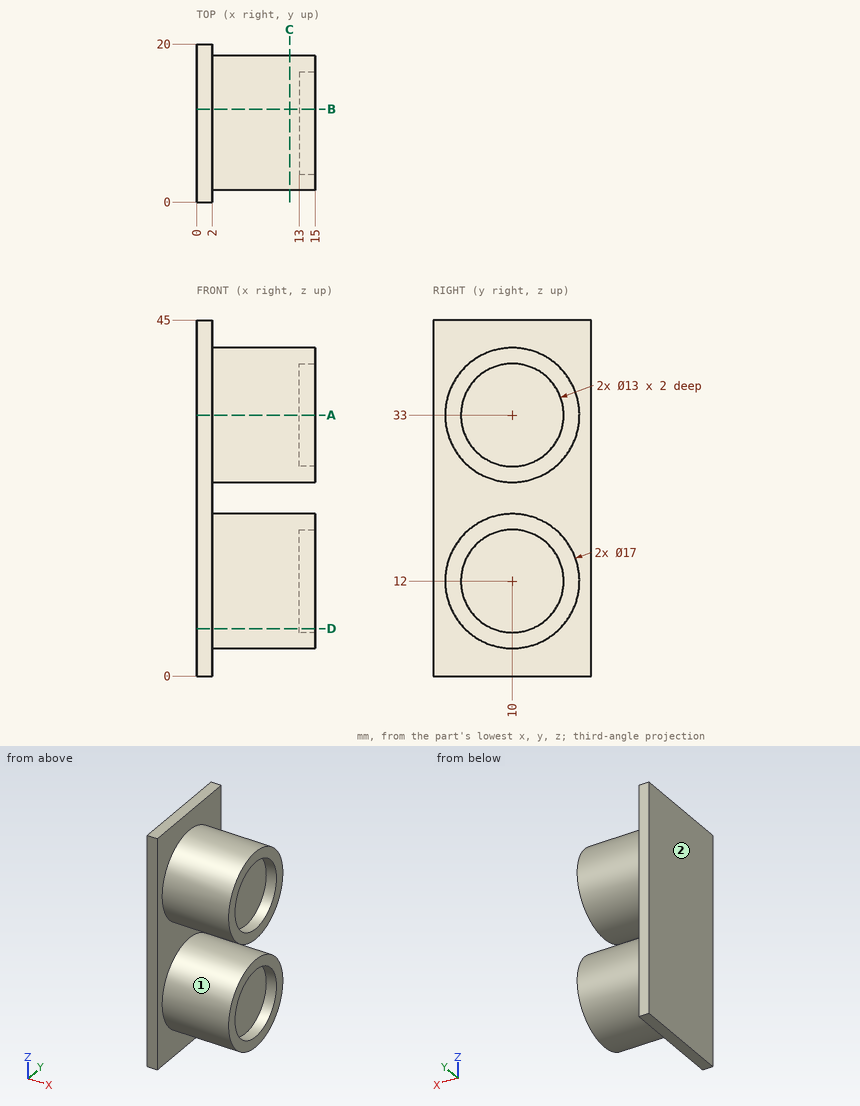
The drawing under review shows one solid part. Ordinate dimensions are in mm from its lowest x, y, z. Give positions to 0.01 mm unless a question says otherwise; leave off trailing zeros. Order: outer loops, then holes, each group sorted by start corner. A loop starts at its lowest first (then second) coordinate and runs counter-clockwise, first axis right, second up. Notation, with made-up numbers: (63, 53) - (84, 53) arc R19 ccw to (84, 78) - close; hole circle Ø11 at (78, 62). An arc over 180 degrees is marked (long way). Answer as a JSON object with one key per item and string values. Group by question number.
Item 1: Take a section at C-C on x = 11.75. Give the boundary of the cut face in (y, z).
Item 2: Wall thickness on line 1 along Y through (x, z) = (13.5, 33); line 2 along X through (y, z) = (11.5, 15.5); line 3 along Z through (x, y) = (7.5, 3.5): over which ranges is each line inside the solid? List them lowest first.
Item 3: Take a section at B-B on y = 11.75. Give the boundary of the cut face in (x, z).
Item 4: Draft analysis for pull direction Z (two halves, no side actions). For the marked faces 1 and 2, state which applies: pulls with the +Z half, pulls with the -Z half, needs draft (parallel to the pull), parting line crosses it, or undercut.
Item 5: Clearance check with flat-ended pins moving along their axes: pin 1 Ø4 at (y, z) = (11, 14.5) entering from +X; pin 2 Ø6 at (x, y) = (7, 14.5) entering from +Z; pin 3 Ø1.5 at (x, y) = (8.5, 10) entering from +Z. State where each tip first meets the part, or that it passes through.
Item 6: Take a section at A-A on z = 33. Give the boundary of the cut face in (x, y), and give its area (3 significant figures).
Item 7: Take a section at D-D on z = 6. Give the boundary of the cut face in (x, y).
Reported:
{
 "1": {"outline": "circle Ø17 at (10, 12); circle Ø17 at (10, 33)"},
 "2": {"line 1": "1.5 to 3.5, 16.5 to 18.5", "line 2": "0 to 13", "line 3": "6.52 to 17.48, 27.52 to 38.48"},
 "3": {"outline": "(0, 0) - (2, 0) - (2, 3.68) - (15, 3.68) - (15, 5.74) - (13, 5.74) - (13, 18.26) - (15, 18.26) - (15, 20.32) - (2, 20.32) - (2, 24.68) - (15, 24.68) - (15, 26.74) - (13, 26.74) - (13, 39.26) - (15, 39.26) - (15, 41.32) - (2, 41.32) - (2, 45) - (0, 45) - close"},
 "4": {"face 1": "undercut", "face 2": "needs draft"},
 "5": {"pin 1": "x = 13", "pin 2": "z = 41.37", "pin 3": "z = 41.5"},
 "6": {"outline": "(0, 0) - (2, 0) - (2, 1.5) - (15, 1.5) - (15, 3.5) - (13, 3.5) - (13, 16.5) - (15, 16.5) - (15, 18.5) - (2, 18.5) - (2, 20) - (0, 20) - close", "area": "235 mm^2"},
 "7": {"outline": "(0, 0) - (2, 0) - (2, 3.98) - (15, 3.98) - (15, 7.5) - (13, 7.5) - (13, 12.5) - (15, 12.5) - (15, 16.02) - (2, 16.02) - (2, 20) - (0, 20) - close"}
}
